Part model, mm, in its own coordinate system. Face numbers are marked on the shaded views. A direction names the side the tool comes from. Round coordinates to 2 decimals unless told otherwise and drop trailing zeros. Order: outer loops, then holes, each group sorted by start corner. A loop starts at its lowest first (then second) coordinate and runs counter-clockwise, first axis right, second up. Notation, with made-up numbers: (48, -16) -> (104, -16) arc R18 ccw to (104, 18) -> close; hole circle Ø11 at (70, 16). An arc over 180 degrees is marked (long way). Use CSV: the item, a comma, the result in double quotes.
```python
from build123d import *

# Parameters (mm, degrees)
CROQUIS1_W                          = 10
CROQUIS1_H                          = 7.7
SALIENTE_EXTRUIR1_DEPTH             = 6.6
SALIENTE_EXTRUIR2_REACH             = 11.131
SALIENTE_EXTRUIR2_DIRECTION_2_REACH = 11.131
CROQUIS3_R                          = 1.85
CORTAR_EXTRUIR1_DEPTH               = 2.2
CORTAR_EXTRUIR2_DEPTH               = 0.25
MATRIZL1_COUNT                      = 2
MATRIZL1_PITCH                      = 5.2
CROQUIS5_W                          = 4.3
CROQUIS5_H                          = 5.4
CROQUIS5_R                          = 0.75
CORTAR_EXTRUIR3_DEPTH               = 0.7
CROQUIS5_2_R                        = 0.75
CORTAR_EXTRUIR4_DEPTH               = 1.2
MATRIZL2_COUNT                      = 2
MATRIZL2_PITCH                      = 5.2
CROQUIS6_R                          = 0.25
SALIENTE_EXTRUIR3_DEPTH             = 6
REDONDEO1_R                         = 0.25


with BuildPart() as part:
    # Croquis1 → Saliente-Extruir1 (new body)
    with BuildSketch(Plane(origin=(0, 0, 0), x_dir=(1, 0, 0), z_dir=(0, 1, 0))):
        Rectangle(CROQUIS1_W, CROQUIS1_H)
    extrude(amount=SALIENTE_EXTRUIR1_DEPTH)

    # Saliente-Extruir2: up to this face of the body (flat: up to its plane)
    saliente_extruir2_end = Plane(part.part.faces().sort_by_distance((5, 3.3, 0))[0])
    # Croquis2 → Saliente-Extruir2 (add, up to the picked face)
    with BuildSketch(Plane(origin=(0, 0, 0), x_dir=(0, 0, -1), z_dir=(1, 0, 0)), mode=Mode.PRIVATE) as saliente_extruir2_sk1:
        Polygon((-3.85, 6.6), (3.85, 6.6), (2.45, 10), (-3.05, 10), align=None)
    saliente_extruir2_tool1 = split(extrude(saliente_extruir2_sk1.sketch, amount=SALIENTE_EXTRUIR2_REACH, mode=Mode.PRIVATE), bisect_by=saliente_extruir2_end, keep=Keep.BOTH, mode=Mode.PRIVATE)
    add(saliente_extruir2_tool1.solids().sort_by(Axis((0, 8.205556, 0.141667), (1, 0, 0)))[0])

    # Saliente-Extruir2 direction 2: up to this face of the body (flat: up to its plane)
    saliente_extruir2_direction_2_end = Plane(part.part.faces().sort_by_distance((-5, 3.3, 0))[0])
    # Croquis2 → Saliente-Extruir2 direction 2 (add, up to the picked face)
    with BuildSketch(Plane(origin=(0, 0, 0), x_dir=(0, 0, -1), z_dir=(1, 0, 0)), mode=Mode.PRIVATE) as saliente_extruir2_direction_2_sk1:
        Polygon((-3.85, 6.6), (3.85, 6.6), (2.45, 10), (-3.05, 10), align=None)
    saliente_extruir2_direction_2_tool1 = split(extrude(saliente_extruir2_direction_2_sk1.sketch, amount=-SALIENTE_EXTRUIR2_DIRECTION_2_REACH, mode=Mode.PRIVATE), bisect_by=saliente_extruir2_direction_2_end, keep=Keep.BOTH, mode=Mode.PRIVATE)
    add(saliente_extruir2_direction_2_tool1.solids().sort_by(Axis((0, 8.205556, 0.141667), (-1, 0, 0)))[0])

    # Croquis3 → Cortar-Extruir1 (cut)
    with BuildSketch(Plane(origin=(0, 10, 0), x_dir=(1, 0, 0), z_dir=(0, 1, 0))):
        with Locations(Location((-2.45, 0, 0), (0, 0, 270))):
            Circle(CROQUIS3_R)
    cortar_extruir1 = extrude(amount=-CORTAR_EXTRUIR1_DEPTH, mode=Mode.SUBTRACT)

    # Croquis4 → Cortar-Extruir2 (cut)
    with BuildSketch(Plane(origin=(0, 7.8, 0), x_dir=(1, 0, 0), z_dir=(0, 1, 0))):
        with BuildLine():
            ThreePointArc((-2.7, -1.833030278), (-2.45, -1.85), (-2.2, -1.833030278))
            Line((-2.2, -1.833030278), (-2.2, -0.25))
            Line((-2.2, -0.25), (-0.616969722, -0.25))
            ThreePointArc((-0.616969722, -0.25), (-0.604247306, -0.125287641), (-0.6, 0))
            ThreePointArc((-0.6, 0), (-0.604247306, 0.125287641), (-0.616969722, 0.25))
            Line((-0.616969722, 0.25), (-2.2, 0.25))
            Line((-2.2, 0.25), (-2.2, 1.833030278))
            ThreePointArc((-2.2, 1.833030278), (-2.45, 1.85), (-2.7, 1.833030278))
            Line((-2.7, 1.833030278), (-2.7, 0.25))
            Line((-2.7, 0.25), (-4.283030278, 0.25))
            ThreePointArc((-4.283030278, 0.25), (-4.3, 0), (-4.283030278, -0.25))
            Line((-4.283030278, -0.25), (-2.7, -0.25))
            Line((-2.7, -0.25), (-2.7, -1.833030278))
        make_face()
    cortar_extruir2 = extrude(amount=-CORTAR_EXTRUIR2_DEPTH, mode=Mode.SUBTRACT)

    # MatrizL1: Cortar-Extruir1, Cortar-Extruir2 ×2
    with Locations(*[(i * MATRIZL1_PITCH, 0, 0) for i in range(1, MATRIZL1_COUNT)]):
        add(cortar_extruir1, mode=Mode.SUBTRACT)
        add(cortar_extruir2, mode=Mode.SUBTRACT)

    # Croquis5 → Cortar-Extruir3 (cut)
    with BuildSketch(Plane.XY.offset(3.85)):
        with Locations((-2.55, 3)):
            Rectangle(CROQUIS5_W, CROQUIS5_H)
        with Locations((-2.55, 2.25)):
            Circle(CROQUIS5_R, mode=Mode.SUBTRACT)
    cortar_extruir3 = extrude(amount=-CORTAR_EXTRUIR3_DEPTH, mode=Mode.SUBTRACT)

    # Croquis5_2 → Cortar-Extruir4 (cut)
    with BuildSketch(Plane.XY.offset(3.85)):
        with Locations((-2.55, 2.25)):
            Circle(CROQUIS5_2_R)
    cortar_extruir4 = extrude(amount=-CORTAR_EXTRUIR4_DEPTH, mode=Mode.SUBTRACT)

    # MatrizL2: Cortar-Extruir3, Cortar-Extruir4 ×2
    with Locations(*[(i * MATRIZL2_PITCH, 0, 0) for i in range(1, MATRIZL2_COUNT)]):
        add(cortar_extruir3, mode=Mode.SUBTRACT)
        add(cortar_extruir4, mode=Mode.SUBTRACT)

    # Croquis6 → Saliente-Extruir3 (add)
    with BuildSketch(Plane.XZ):
        with Locations(Location((2.45, 0, 0), (0, 0, 90))):
            Circle(CROQUIS6_R)
        with Locations(Location((-2.45, 0, 0), (0, 0, 90))):
            Circle(CROQUIS6_R)
    extrude(amount=SALIENTE_EXTRUIR3_DEPTH)

    # Redondeo1
    redondeo1_edges = [part.edges().sort_by_distance(p)[0] for p in [
        (2.45, -6, -0.25),
        (-2.45, -6, -0.25),
    ]]
    fillet(redondeo1_edges, radius=REDONDEO1_R)


solid = part.part
```
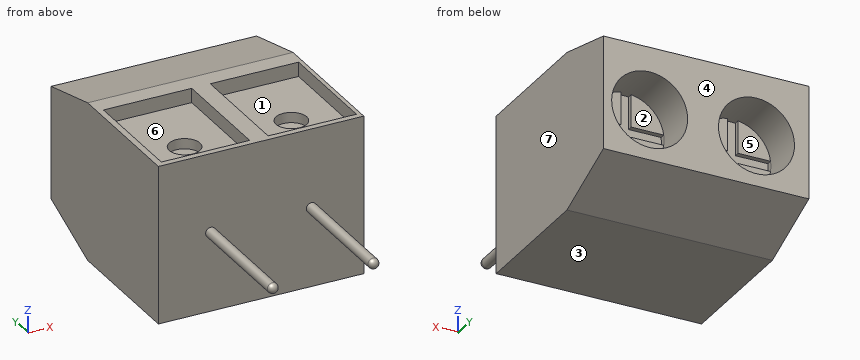
(1) Drop flat-ended pins along their axis: P1, Ø1.3, axis at x = 2, y = 4, coming from the +Z side; P2, Ø4, axis at x = 0, z = 0.5, coming from the -Y side. Give the stop position or say it passes through.
Reply:
P1,"z = 3.15"
P2,"y = 0"
(2) Cut at C-C, the plane y = 2.25. Give the cut face in (x, z).
Reply:
outline,"(-5, -3.85) -> (5, -3.85) -> (5, 3.85) -> (4.8, 3.85) -> (4.8, 3.15) -> (3.4, 3.15) -> (3.4, 2.65) -> (1.9, 2.65) -> (1.9, 3.15) -> (0.5, 3.15) -> (0.5, 3.85) -> (-0.4, 3.85) -> (-0.4, 3.15) -> (-1.8, 3.15) -> (-1.8, 2.65) -> (-3.3, 2.65) -> (-3.3, 3.15) -> (-4.7, 3.15) -> (-4.7, 3.85) -> (-5, 3.85) -> close"
(3) Probe probe 1 along X at (y, z) = (9.25, 0); probe 2 along X at (y, z) = (-2, 0); probe 3 along Y at (x, z) = (-2.55, 3). List the from-to ranges inside material, lowest first. Write a range as [from, to].
Reply:
probe 1,"[-5, -4.3], [-0.6, 0.9], [4.6, 5]"
probe 2,"[-2.7, -2.2], [2.2, 2.7]"
probe 3,"[0, 1.5], [3, 10]"
(4) Which spindle directions (+Z, -Z, +X, -X, +Y, -Y) get a long thin tool onto all of the face, cutting with end or side? Do the marked faces 1, 2 and 3. Say none if no direction does.
Reply:
face 1,"+Z"
face 2,"+Y"
face 3,"-Z, +X, -X, +Y, -Y"
(5) Cut at A-A, the plane y = 4.25. Give the cut face in (x, z).
Reply:
outline,"(-5, -3.85) -> (5, -3.85) -> (5, 3.85) -> (4.8, 3.85) -> (4.8, 3.15) -> (0.5, 3.15) -> (0.5, 3.85) -> (-0.4, 3.85) -> (-0.4, 3.15) -> (-4.7, 3.15) -> (-4.7, 3.85) -> (-5, 3.85) -> close"
(6) Cut at B-B, the plane z = -0.5. Give the cut face in (x, y).
Reply:
outline,"(-5, 0) -> (5, 0) -> (5, 10) -> (4.53, 10) -> (4.53, 7.8) -> (3, 7.8) -> (3, 7.55) -> (2.5, 7.55) -> (2.5, 7.8) -> (0.97, 7.8) -> (0.97, 10) -> (-0.67, 10) -> (-0.67, 7.8) -> (-2.2, 7.8) -> (-2.2, 7.55) -> (-2.7, 7.55) -> (-2.7, 7.8) -> (-4.23, 7.8) -> (-4.23, 10) -> (-5, 10) -> close"
(7) Pull direction X, two halves, no side cores. Call the marked faces 4, 5, 6 and 7: released by +X, released by -X, zero draft, split by the parting line, or undercut.
Reply:
face 4,"zero draft"
face 5,"undercut"
face 6,"undercut"
face 7,"released by +X"
(8) Cut at D-D, the plane x = -1. Give the cut face in (y, z), then the cut area to 3 significant figures.
Reply:
outline,"(0, -3.85) -> (6.6, -3.85) -> (10, -2.45) -> (10, -1.15) -> (7.8, -1.15) -> (7.8, -0.25) -> (7.55, -0.25) -> (7.55, 0.25) -> (7.8, 0.25) -> (7.8, 1.15) -> (10, 1.15) -> (10, 3.05) -> (6.6, 3.85) -> (5.7, 3.85) -> (5.7, 3.15) -> (0.3, 3.15) -> (0.3, 3.85) -> (0, 3.85) -> close"
area,"64.3 mm2"
